Check sheet for the drawn part. Datum: minimum x, y, z corner. Units: mm. A direction names the side the tool comes from. Coordinates: 2 decimals unless noted, no trailing zeros. Loops run counter-clockwise (first coordinate to the right, second up) from the corner with the lowest first, then second, coordinate; pieces in that order, holes last. Notation, with made-up numbers: (19.5, 84) -> (51.5, 84) arc R14 ccw to (51.5, 91) -> close; hole circle Ø7 at (28.25, 9). An arc over 180 degrees is marked (long way). Use CSV: the item, a comma, the result in double quotes. Start each with the question number.
1. Sectioned sample at B-B, the plane x = 5.75. Record the cut outline in (y, z).
2. Sectioned sample at C-C, the plane z = 3. Record the cut outline in (x, y), and give its area (3 significant figures).
3. Sectioned sample at D-D, the plane y = 1.25. Record the cut outline in (x, z), and give its area (3 significant figures).
4. Gauge pin test, flat ends, axial feed: pin 1 (0.6 mm diameter, centred on y = 3, z = 5, fed in from -X); pin 2 (1.6 mm diameter, centred on x = 5.5, z = 6, fed in from +Y); pin 3 (4 mm diameter, centred on x = 1.5, y = 8.5, fed in from +Z); pin 4 (1.8 mm diameter, centred on x = 5, y = 5, fed in from +Z). Record the tip position at first contact, or that the pin passes through.
5. Sectioned sample at A-A, the plane y = 5. Record the cut outline in (x, z), and give its area (3 significant figures).
6. Set-up check for the marked faces 1, 2 and 3: record each of +Z, -Z, +X, -X, +Y, -Y from which the full face is reachable in a straight line by a thin tool's end or side.
7. Thickness scan on L1, parallel to Y at x = 5, z = 1.5; L2, parallel to X at y = 5, z = 3. Record the ranges inside material, lowest first.
8. Release check for a two-part mould opening along Y. For the marked faces 4, 5, 6 and 7 record: pulls with the +Y half, pulls with the -Y half, needs draft (parallel to the pull), parting line crosses it, or undercut.
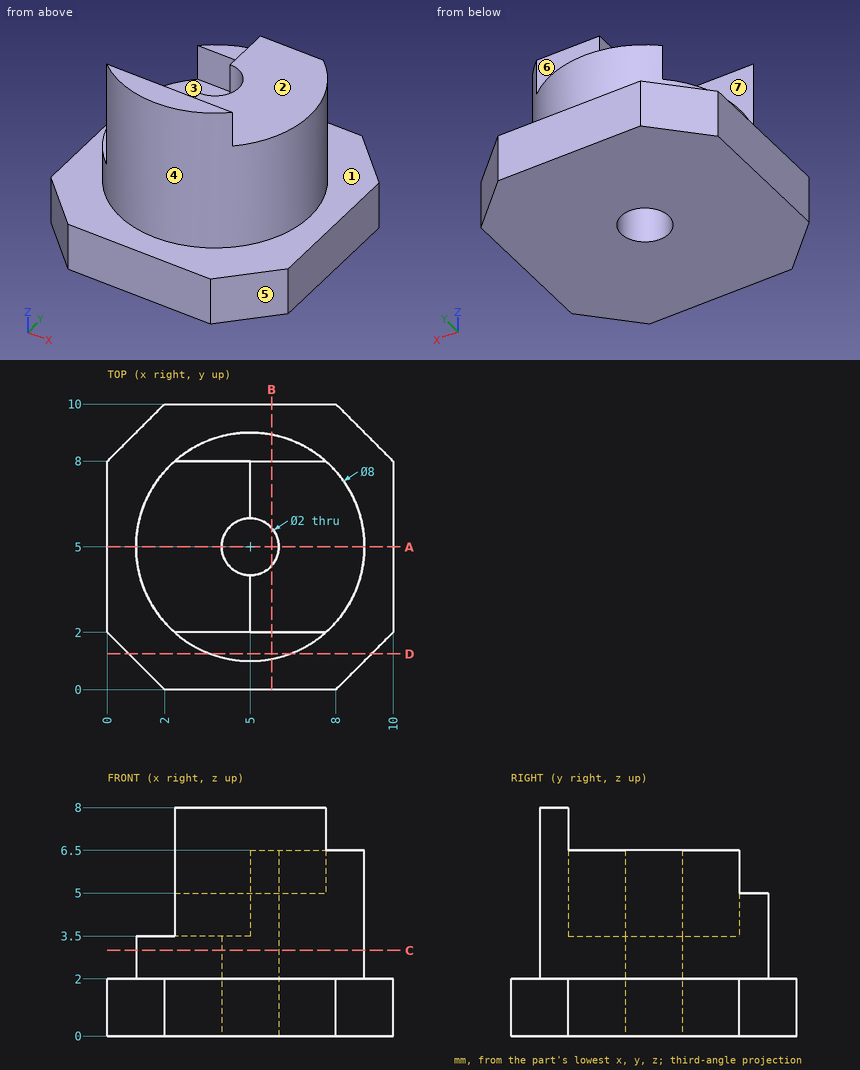
Completed:
1,outline,"(0, 0) -> (4.34, 0) -> (4.34, 6.5) -> (2, 6.5) -> (2, 8) -> (1.07, 8) -> (1.07, 2) -> (0, 2) -> close; (5.66, 0) -> (10, 0) -> (10, 2) -> (8.93, 2) -> (8.93, 5) -> (8, 5) -> (8, 6.5) -> (5.66, 6.5) -> close"
2,outline,"circle Ø8 at (5, 5); hole circle Ø2 at (5, 5)"
2,area,"47.1 mm²"
3,outline,"(0.75, 0) -> (9.25, 0) -> (9.25, 2) -> (6.39, 2) -> (6.39, 8) -> (3.61, 8) -> (3.61, 2) -> (0.75, 2) -> close"
3,area,"33.7 mm²"
4,pin 1,"x = 5"
4,pin 2,"y = 8"
4,pin 3,"z = 5"
4,pin 4,"through"
5,outline,"(0, 0) -> (4, 0) -> (4, 3.5) -> (1, 3.5) -> (1, 2) -> (0, 2) -> close; (6, 0) -> (10, 0) -> (10, 2) -> (9, 2) -> (9, 6.5) -> (6, 6.5) -> close"
5,area,"34.0 mm²"
6,face 1,"+Z"
6,face 2,"+Z, +X, -X, +Y"
6,face 3,"+Z, -X"
7,L1,"0 to 4, 6 to 10"
7,L2,"1 to 4, 6 to 9"
8,face 4,"parting line crosses it"
8,face 5,"pulls with the -Y half"
8,face 6,"pulls with the +Y half"
8,face 7,"undercut"
